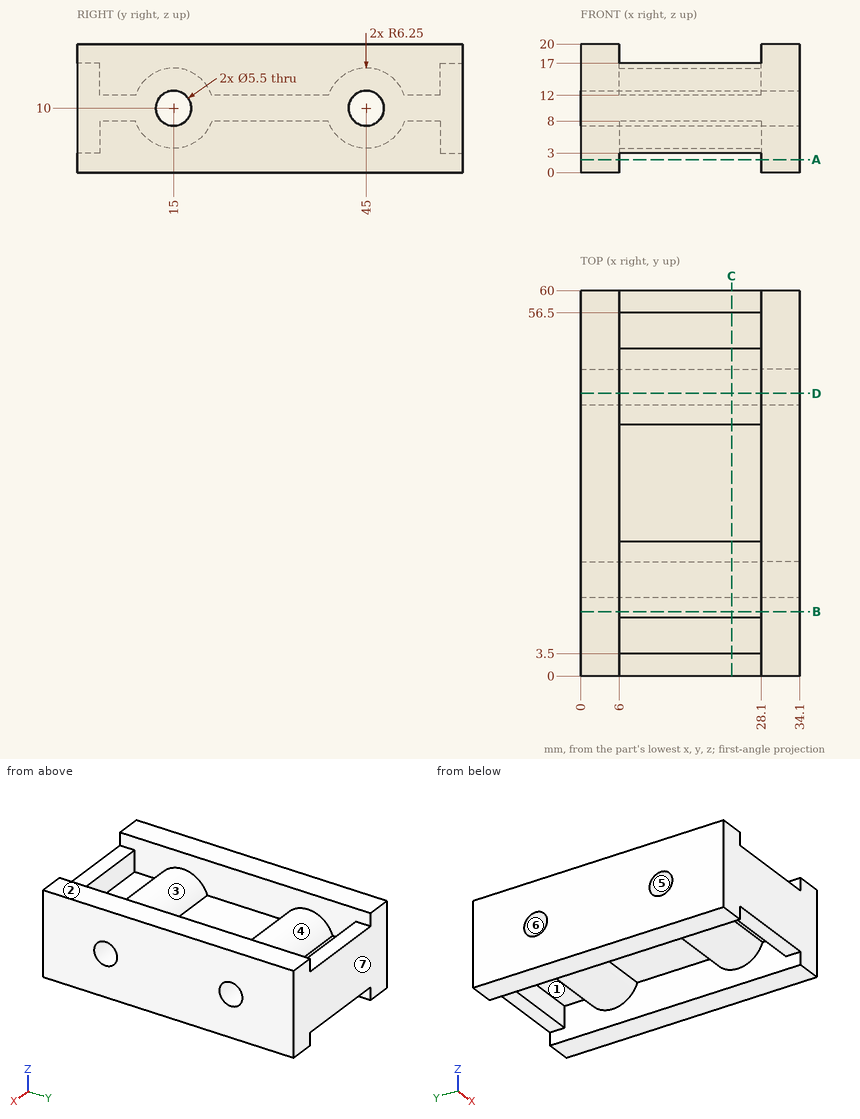
Here's the drawing with two shaded views (mm, measured from the low corner). I have some questions. A direction names the side the tool comes from. Give positions to 0.01 mm unless a question says otherwise; leave off trailing zeros. Write each loop counter-clockwise with the first axis right and the second up, starting at its lowest first coordinate (ties: lowest second). Pieces come first, ordered by that corner, then holes. Notation, with made-up numbers: (-24, -10.75) - (9, -10.75) arc R21 cw to (9, 4.25) - close; hole circle Ø5 at (-10.75, 78). An arc over 180 degrees is marked (long way). Write item = value, one per line. Start each with the question number.
1. Imagine slicing it at A-A (z = 2). Please give me the cut outline in (x, y).
2. Please list where these lines run through material, in increasing order: line 1 (Y direction, x = 20, z = 10); line 2 (X direction, y = 17, z = 18.25); line 3 (Y direction, x = 25.5, z = 11.5).
3. Imagine slicing it at C-C (x = 23.5). Please give me the cut outline in (y, z).
4. Thinking about a two-plate mould opening in Z: for the marked faces 4, 5, 6 and 7, which applies, released by +Z, released by -Z, zero draft, split by the parting line, or undercut?
5. For pin 1 (2.5 mm diameter, centred on x = 20, z = 14, fed in from -Y); pin 2 (6 mm diameter, centred on x = 21, y = 53, fed in from +Z); pin 3 (4.5 mm diameter, centred on x = 16.5, y = 6, fed in from +Z); pin 4 (4 mm diameter, centred on x = 21, y = 58, fed in from +Z), each with a flat end and sliding along its axis, tell me the tip position at first contact or that it passes through.
6. Imagine slicing it at D-D (y = 44). Please give me the cut outline in (x, z), and give its area (3 significant figures).
7. Imagine slicing it at B-B (y = 10). Please give me the cut outline in (x, z), and give its area (3 significant figures).
8. On a 3-axis mill with a long thin cutter (end or side, diameter ignored), from which of +Z, -Z, +X, -X, +Y, -Y can I reach the whole of each face in a straight line? I mean the marked faces 1, 2 and 3. Say none if no direction works.
Worked answers:
q1.outline = (0, 0) - (6, 0) - (6, 60) - (0, 60) - close; (28.1, 0) - (34.1, 0) - (34.1, 60) - (28.1, 60) - close
q2.line_1 = 0 to 12.25, 17.75 to 42.25, 47.75 to 60
q2.line_2 = 0 to 6, 28.1 to 34.1
q2.line_3 = 0 to 12.7, 17.3 to 42.7, 47.3 to 60
q3.outline = (0, 3) - (3.5, 3) - (3.5, 8) - (9.08, 8) arc R6.25 ccw to (20.92, 8) - (39.08, 8) arc R6.25 ccw to (50.92, 8) - (56.5, 8) - (56.5, 3) - (60, 3) - (60, 17) - (56.5, 17) - (56.5, 12) - (50.92, 12) arc R6.25 ccw to (39.08, 12) - (20.92, 12) arc R6.25 ccw to (9.08, 12) - (3.5, 12) - (3.5, 17) - (0, 17) - close; hole circle Ø5.5 at (15, 10); hole circle Ø5.5 at (45, 10)
q4.face_4 = released by +Z
q4.face_5 = undercut
q4.face_6 = undercut
q4.face_7 = zero draft
q5.pin_1 = 0
q5.pin_2 = 13.75
q5.pin_3 = 12
q5.pin_4 = 17
q6.outline = (0, 0) - (6, 0) - (6, 3.83) - (28.1, 3.83) - (28.1, 0) - (34.1, 0) - (34.1, 7.44) - (0, 7.44) - close; (0, 12.56) - (34.1, 12.56) - (34.1, 20) - (28.1, 20) - (28.1, 16.17) - (6, 16.17) - (6, 20) - (0, 20) - close
q6.area = 338 mm2
q7.outline = (0, 0) - (6, 0) - (6, 6.25) - (28.1, 6.25) - (28.1, 0) - (34.1, 0) - (34.1, 20) - (28.1, 20) - (28.1, 13.75) - (6, 13.75) - (6, 20) - (0, 20) - close
q7.area = 406 mm2
q8.face_1 = -Z
q8.face_2 = +Z, +X, -X, +Y, -Y
q8.face_3 = +Z
